from build123d import *

# Parameters (mm, degrees)
PAD_DEPTH       = 1
SKETCH001_W     = 12
SKETCH001_H     = 12
PAD001_DEPTH    = 1
SKETCH002_W     = 12
SKETCH002_H     = 14
PAD002_DEPTH    = 0.5
SKETCH003_W     = 12
SKETCH003_H     = 12
PAD003_DEPTH    = 1.5
PAD004_DEPTH    = 4
SKETCH005_W     = 8
SKETCH005_H     = 4
POCKET_DEPTH    = 0.2
PAD005_DEPTH    = 0.2
SKETCH007_W     = 2
SKETCH007_H     = 6
PAD006_DEPTH    = 0.2
SKETCH008_R     = 0.5
POCKET001_DEPTH = 0.2
SKETCH009_W     = 3.383523
SKETCH009_H     = 4.158913
PAD007_DEPTH    = 0.2
PAD008_DEPTH    = 0.2
SKETCH011_W     = 0.321104
SKETCH011_H     = 4.367
PAD009_DEPTH    = 3
PAD010_DEPTH    = 0.2
SKETCH013_W     = 2
SKETCH013_H     = 6
PAD011_DEPTH    = 4
SKETCH014_W     = 6
SKETCH014_H     = 10
PAD012_DEPTH    = 0.2
PAD013_DEPTH    = 0.2
SKETCH016_W     = 2.5
SKETCH016_H     = 2.8
PAD014_DEPTH    = 6
SKETCH018_W     = 1.2
SKETCH018_H     = 1.5
POCKET002_DEPTH = 0.5
SKETCH019_W     = 2
SKETCH019_H     = 2.8
POCKET003_DEPTH = 0.1
SKETCH020_W     = 0.738537
SKETCH020_H     = 1.573408
PAD015_DEPTH    = 0.8
SKETCH021_W     = 1.524805
SKETCH021_H     = 0.946431
PAD016_DEPTH    = 0.1
POCKET004_DEPTH = 5
SKETCH023_W     = 1.745958
SKETCH023_H     = 0.71265
POCKET005_DEPTH = 0.1
SKETCH024_W     = 6.7
SKETCH024_H     = 6.33
PAD017_DEPTH    = 2
SKETCH025_W     = 0.3
SKETCH025_H     = 6
PAD018_DEPTH    = 2
SKETCH026_W     = 7.882242
SKETCH026_H     = 3.90727
PAD019_DEPTH    = 2
POCKET006_DEPTH = 1.5
FILLET_R        = 1
PAD020_DEPTH    = 0.1


with BuildPart() as part:
    # Sketch → Pad (new body)
    with BuildSketch(Plane.XY):
        Polygon((0, -28), (-40, -28), (-40, 0), (-16, 0), (-16, 12), (12, 12), (12, -24), (0, -24), align=None)
    extrude(amount=PAD_DEPTH)

    # Sketch001 (on Face10 of Pad) → Pad001 (join)
    with BuildSketch(Plane.XY.offset(1)):
        with Locations((6, 6)):
            Rectangle(SKETCH001_W, SKETCH001_H)
    extrude(amount=PAD001_DEPTH)

    # Sketch002 (on Face5 of Pad001) → Pad002 (join)
    with BuildSketch(Plane.XY.offset(1)):
        with Locations((6, -7)):
            Rectangle(SKETCH002_W, SKETCH002_H)
    extrude(amount=PAD002_DEPTH)

    # Sketch003 (on Face5 of Pad002) → Pad003 (join)
    with BuildSketch(Plane.XY.offset(1)):
        with Locations((-6, 6)):
            Rectangle(SKETCH003_W, SKETCH003_H)
    extrude(amount=PAD003_DEPTH)

    # Sketch004 (on Face8 of Pad003) → Pad004 (join)
    with BuildSketch(Plane(origin=(-16, 0, 0), x_dir=(0, -1, 0), z_dir=(-1, 0, 0))):
        Polygon((-12, 0), (-12, 1), (-9, 1), (-9, 2.1249999998), (-8.1428571429, 2.1249999998), (-8.1428571429, 3.2499999997), (-7.2857142857, 3.2499999997), (-7.2857142857, 4.3749999997), (-6.4285714286, 4.3749999997), (-6.4285714286, 5.4999999997), (-5.5714285714, 5.4999999997), (-5.5714285714, 6.6249999997), (-4.7142857143, 6.6249999997), (-4.7142857143, 7.7499999998), (-3.8571428571, 7.7499999998), (-3.8571428571, 8.8749999999), (-3, 8.8749999999), (-3, 10), (0, 10), (0, 0), align=None)
    extrude(amount=-PAD004_DEPTH)

    # Sketch005 (on Face29 of Pad004) → Pocket (cut)
    with BuildSketch(Plane.XY.offset(2)):
        with Locations((7.8244701681, 9.794484)):
            Rectangle(SKETCH005_W, SKETCH005_H)
    extrude(amount=-POCKET_DEPTH, mode=Mode.SUBTRACT)

    # Sketch006 (on Face29 of Pocket) → Pad005 (join)
    with BuildSketch(Plane.XY.offset(2)):
        with BuildLine():
            ThreePointArc((7, 0), (6.1213203436, 2.1213203436), (4, 3))
            Line((4, 3), (4, 0))
            Line((4, 0), (7, 0))
        make_face()
    extrude(amount=PAD005_DEPTH)

    # Sketch007 (on Face29 of Pad005) → Pad006 (join)
    with BuildSketch(Plane.XY.offset(2)):
        with Locations((10.75453, 3.2614561845)):
            Rectangle(SKETCH007_W, SKETCH007_H)
    extrude(amount=PAD006_DEPTH)

    # Sketch008 (on Face58 of Pad006) → Pocket001 (cut)
    with BuildSketch(Plane.XY.offset(2.2)):
        with Locations((10.739349, 5.010931)):
            Circle(SKETCH008_R)
        with Locations((10.739349, 1.739257)):
            Circle(SKETCH008_R)
    extrude(amount=-POCKET001_DEPTH, mode=Mode.SUBTRACT)

    # Sketch009 (on Face29 of Pocket001) → Pad007 (join)
    with BuildSketch(Plane.XY.offset(2)):
        with Locations((1.8727195, 9.8045235)):
            Rectangle(SKETCH009_W, SKETCH009_H)
    extrude(amount=PAD007_DEPTH)

    # Sketch010 (on Face29 of Pad007) → Pad008 (join)
    with BuildSketch(Plane.XY.offset(2)):
        with BuildLine():
            ThreePointArc((2.40198, 3.464925), (1.876188, 3.990717), (1.350396, 3.464925))
            Line((1.350396, 3.464925), (1.350396, 1.572068))
            ThreePointArc((1.350396, 1.572068), (1.876188, 1.046276), (2.40198, 1.572068))
            Line((2.40198, 3.464925), (2.40198, 1.572068))
        make_face()
    extrude(amount=PAD008_DEPTH)

    # Sketch011 (on Face29 of Pad008) → Pad009 (join)
    with BuildSketch(Plane.XY.offset(2)):
        with Locations((3.379871, 2.379998)):
            Rectangle(SKETCH011_W, SKETCH011_H)
    extrude(amount=PAD009_DEPTH)

    # Sketch012 (on Face29 of Pad009) → Pad010 (join)
    with BuildSketch(Plane.XY.offset(2)):
        with BuildLine():
            ThreePointArc((0.0127659439, 4.2328060849), (2.1340862875, 5.1114857414), (3.0127659439, 7.2328060849))
            Line((3.0127659439, 7.2328060849), (0.0127659439, 7.2328060849))
            Line((0.0127659439, 7.2328060849), (0.0127659439, 4.2328060849))
        make_face()
    extrude(amount=PAD010_DEPTH)

    # Sketch013 (on Face5 of Pad010) → Pad011 (join)
    with BuildSketch(Plane.XY.offset(1)):
        with Locations((4.6129902875, -17.0670078745)):
            Rectangle(SKETCH013_W, SKETCH013_H)
    extrude(amount=PAD011_DEPTH)

    # Sketch014 (on Face5 of Pad011) → Pad012 (join)
    with BuildSketch(Plane.XY.offset(1)):
        with Locations((8.8879963878, -18.9493321845)):
            Rectangle(SKETCH014_W, SKETCH014_H)
    extrude(amount=PAD012_DEPTH)

    # Sketch015 (on Face29 of Pad012) → Pad013 (join)
    with BuildSketch(Plane.XY.offset(1.5)):
        with BuildLine():
            ThreePointArc((0.0906927099, -7.9815394859), (2.2120130535, -7.1028598295), (3.0906927099, -4.9815394859))
            Line((3.0906927099, -4.9815394859), (0.0906927099, -4.9815394859))
            Line((0.0906927099, -4.9815394859), (0.0906927099, -7.9815394859))
        make_face()
    extrude(amount=PAD013_DEPTH)

    # Sketch016 (on Face5 of Pad013) → Pad014 (join)
    with BuildSketch(Plane.XY.offset(1)):
        with Locations((10.5483907095, -22.2439987125)):
            Rectangle(SKETCH016_W, SKETCH016_H)
    extrude(amount=PAD014_DEPTH)

    # Sketch018 (on Face36 of Pad014) → Pocket002 (cut)
    with BuildSketch(Plane.XY.offset(5)):
        with Locations((4.6740733219, -15.2416696781)):
            Rectangle(SKETCH018_W, SKETCH018_H)
    extrude(amount=-POCKET002_DEPTH, mode=Mode.SUBTRACT)

    # Sketch019 (on Face21 of Pocket002) → Pocket003 (cut)
    with BuildSketch(Plane(origin=(3.6129902875, 0, 0), x_dir=(0, -1, 0), z_dir=(-1, 0, 0))):
        with Locations((18.8170917125, 2.5448113219)):
            Rectangle(SKETCH019_W, SKETCH019_H)
    extrude(amount=-POCKET003_DEPTH, mode=Mode.SUBTRACT)

    # Sketch020 (on Face36 of Pocket003) → Pad015 (join)
    with BuildSketch(Plane.XY.offset(5)):
        with Locations((4.7687005, -18.196731)):
            Rectangle(SKETCH020_W, SKETCH020_H)
    extrude(amount=PAD015_DEPTH)

    # Sketch021 (on Face44 of Pad015) → Pad016 (join)
    with BuildSketch(Plane(origin=(0, -20.8439987125, 0), x_dir=(-1, 0, 0), z_dir=(0, 1, 0))):
        with Locations((-10.5244535, 6.0330185)):
            Rectangle(SKETCH021_W, SKETCH021_H)
    extrude(amount=PAD016_DEPTH)

    # Sketch022 (on Face45 of Pad016) → Pocket004 (cut)
    with BuildSketch(Plane.YZ.offset(11.7983907095)):
        Polygon((-20.527332, 3.292079), (-22.183851, 4.155583), (-22.254341, 4.701882), (-20.527332, 5.565385), align=None)
    extrude(amount=-POCKET004_DEPTH, mode=Mode.SUBTRACT)

    # Sketch023 (on Face101 of Pocket004) → Pocket005 (cut)
    with BuildSketch(Plane(origin=(0, -3.0366433765, -5.8254014449), x_dir=(1, 0, 0), z_dir=(0, 0.4622433354, 0.8867531217))):
        with Locations((10.59525, -20.547228)):
            Rectangle(SKETCH023_W, SKETCH023_H)
    extrude(amount=-POCKET005_DEPTH, mode=Mode.SUBTRACT)

    # Sketch024 (on Face29 of Pocket005) → Pad017 (join)
    with BuildSketch(Plane.XY.offset(1.5)):
        with Locations((8.6312609088, -7.1204113075)):
            Rectangle(SKETCH024_W, SKETCH024_H)
    extrude(amount=PAD017_DEPTH)

    # Sketch025 (on Face110 of Pad017) → Pad018 (join)
    with BuildSketch(Plane.XY.offset(3.5)):
        with Locations((11.800813, -6.9834993219)):
            Rectangle(SKETCH025_W, SKETCH025_H)
    extrude(amount=PAD018_DEPTH)

    # Sketch026 (on Face120 of Pad018) → Pad019 (join)
    with BuildSketch(Plane.XY.offset(1.8)):
        with Locations((7.82612, 9.807974)):
            Rectangle(SKETCH026_W, SKETCH026_H)
    extrude(amount=PAD019_DEPTH)

    # Sketch027 (on Face144 of Pad019) → Pocket006 (cut)
    with BuildSketch(Plane.XY.offset(3.8)):
        with BuildLine():
            ThreePointArc((5.903537, 10.860499), (4.754228, 9.71119), (5.903537, 8.561881))
            Line((5.903537, 8.561881), (9.843761, 8.561881))
            ThreePointArc((9.843761, 8.561881), (10.99307, 9.71119), (9.843761, 10.860499))
            Line((5.903537, 10.860499), (9.843761, 10.860499))
        make_face()
    extrude(amount=-POCKET006_DEPTH, mode=Mode.SUBTRACT)

    # Fillet
    fillet_edges = [part.edges().sort_by_distance(p)[0] for p in [
        (7.873649, 10.860499, 2.3),
    ]]
    fillet(fillet_edges, radius=FILLET_R)

    # Sketch017 (on Face5 of Pad014) → Pad020 (join)
    with BuildSketch(Plane.XY.offset(1)):
        with BuildLine():
            ThreePointArc((3.6318966642, -23.8926850513), (2.7504200176, -21.7764964464), (0.6319071596, -20.9006205647))
            Line((0.6319071596, -23.9006205647), (0.6319071596, -20.9006205647))
            Line((3.6318966642, -23.8926850513), (0.6319071596, -23.9006205647))
        make_face()
    extrude(amount=PAD020_DEPTH)


solid = part.part
Here's how the part is built. I have some questions about the finished solid (model axes, mm). A direction names the side the tool comes from. Coordinates: 2 decimals unless noted, no trailing zeros. Order: outer loops, then holes, each group sorted by start corner. A loop starts at its lowest first (then second) coordinate and runs counter-clockwise, first axis right, second up.
Item 1: For faces 1 (the face through (-14, 4.714, 7)), 2 (the face through (7.901, 10.575, 2.601)), 3 (the face through (2, 3, 2.2)), 4 (the face through (-14, 11, 1)), 5 (the face through (5, 1, 2.2)), which set-ups out of +Z, -Z, +X, -X, +Y, -Y let a thin tool reach every point of the face, with its end or its side?
Result sheet:
face 1: +Z, +X, -X, +Y
face 2: +Z
face 3: +Z, +Y, -Y
face 4: +Z, -X, +Y
face 5: +Z, +X
Item 2: If we section it at A-A on x = -4: List the corners of the cut face in (y, z) for me.
Result sheet:
outline: (-28, 0) - (12, 0) - (12, 2.5) - (0, 2.5) - (0, 1) - (-28, 1) - close
Item 3: If we section it at B-B on x = -33: List the corners of the cut face in (y, z) for me.
Result sheet:
outline: (-28, 0) - (0, 0) - (0, 1) - (-28, 1) - close
Item 4: If we mould it in two halves opening along Y, with no side actions, what happens to faces 6 (the face through (9, -7, 3.5)), 7 (the face through (-12, 10, 2)), 8 (the face through (-14, 6.429, 5))? For each: +Y half, -Y half, draft (parallel to the pull), parting line (faces both ways), or undercut.
Result sheet:
face 6: undercut
face 7: draft
face 8: +Y half
Item 5: For P1, Ø4.5, axis at x = 8.5, y = 9.5, coming from the +Z side; P2, Ø3, axis at x = -34.5, z = 3, coming from the +Y side; P3, Ø2.5, axis at y = 2.5, z = 4, coming from the +X side; P4, Ø12, axis at x = -21, y = -22.5, coming from the +Z side, each with a flat end and sliding along its axis, tell me the tip position at first contact or that it passes through.
Result sheet:
P1: stops at z = 3.8
P2: passes through
P3: stops at x = 3.54
P4: stops at z = 1
Item 6: I need wall thicknesses on line 1 (X direction, y = -20, z = 4); line 2 (Y direction, x = -2, z = 2.25); line 3 (Z direction, x = 1, y = -6). Which ranges of each line are inside material? Lowest first, please.
Result sheet:
line 1: x = 3.61 to 5.61
line 2: y = 0 to 12
line 3: z = 0 to 1.7
